Print and shaded views of the part. All mm, measured from the part's lowest x, y and z. Round coordinates to 2 decimals unless told otherwise and drop trailing zeros. Order: outer loops, then holes, each group sorted by start corner. A loop starts at its lowest first (then second) coordinate and runs counter-clockwise, first axis right, second up. Notation, with made-up numbers: (-2.75, 63) - (44.25, 63) arc R24 ccw to (44.25, 76) - close; hole circle Ø8 at (21, 43). An arc over 180 degrees is marked (long way). Return JSON: item names as keys, results as strings. Group by question number.
Item 1: Saw through at C-C on x = 8.5. List the corners of the cut face in (y, z), and give its area (3 significant figures).
Item 2: Two-plate mould, pull along X, no slides. Class the marked faces 1, 2, 3 and 4: released by +X, released by -X, zero draft, split by the parting line, or undercut.
Item 3: Saw through at A-A on y = 25.75. List the corners of the cut face in (x, z), and give its area (3 significant figures).
Item 4: Probe probe 1 along X at (y, z) = (13, 23.5); probe 2 along Y at (x, z) = (38, 16.75). List the from-to ranges inside material, lowest first.
Item 5: Saw through at B-B on z = 19. List the corners of the cut face in (x, y), and give its area (3 significant figures).
Item 6: Drop flat-ended pins along their axis: pin 1 (5 mm diameter, centred on x = 12.5, z = 16.5, fed in from -Y); pin 2 (15 mm diameter, centred on x = 25.5, z = 18.5, fed in from +Y). Give the stop position or say it passes through.
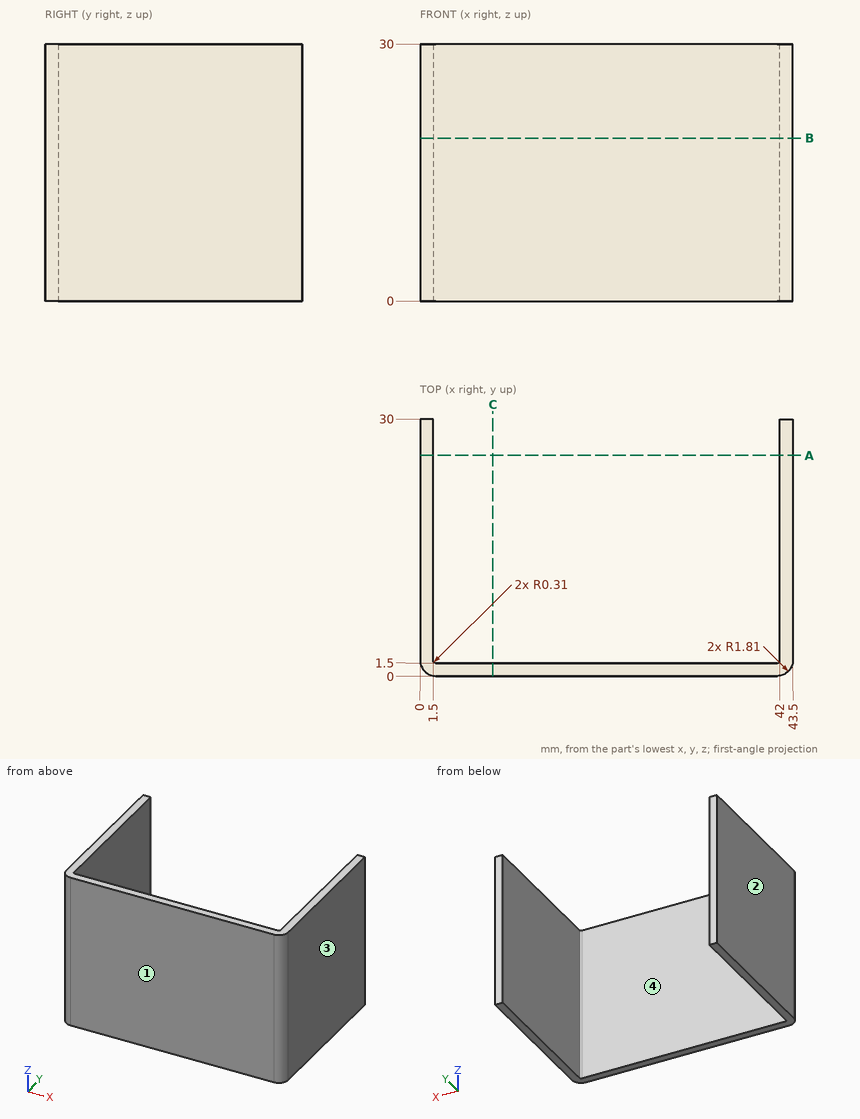
Filled in:
{
 "1": {"outline": "(0, 0) - (1.5, 0) - (1.5, 30) - (0, 30) - close", "area": "45.0 mm^2"},
 "2": {"face 1": "zero draft", "face 2": "released by -X", "face 3": "released by +X", "face 4": "undercut"},
 "3": {"outline": "(0, 0) - (1.5, 0) - (1.5, 30) - (0, 30) - close; (42, 0) - (43.5, 0) - (43.5, 30) - (42, 30) - close", "area": "90.0 mm^2"},
 "4": {"probe 1": "x = 0 to 1.5, 42 to 43.5", "probe 2": "y = 0 to 1.5"},
 "5": {"outline": "(0, 1.81) arc R1.81 ccw to (1.81, 0) - (41.69, 0) arc R1.81 ccw to (43.5, 1.81) - (43.5, 30) - (42, 30) - (42, 1.81) arc R0.31 cw to (41.69, 1.5) - (1.81, 1.5) arc R0.31 cw to (1.5, 1.81) - (1.5, 30) - (0, 30) - close", "area": "149 mm^2"},
 "6": {"pin 1": "stops at y = 0", "pin 2": "stops at y = 1.5"}
}
